The listing builds one solid part. Answer for the finished solid, in the listing's coordinates (mm). Round coordinates to 2 decimals unless told otherwise and drop trailing zeros. Loops run counter-clockwise (first coordinate to the right, second up) from the corner with the lowest first, then second, coordinate; pieces in that order, holes last. Notation, with made-up numbers: (-30.5, 81) -> (-2.5, 81) arc R11 cw to (-2.5, 99) -> close; hole circle Ø11 at (57.5, 35). An arc over 180 degrees is marked (long way). Use a Markdown table: item, result. Add a question column.
Q1. Consider line 1 (Z direction, x = 15.25, y = 19). Determine where the line is inside the solid, lowest interval first.
Q2. For a pull along Y with two mould halves and no side action, classify faces 1 (the flat face through (5, 25, 2)), 2 (the flat face through (9, 0, 1)), 3 (the flat face through (13, 24, 1.9)) as released by +Y, released by -Y, zero draft, split by the parting line, or undercut.
Q3. Section A-A on y = 18.5 is taken. Give the vertices of the cut face in (x, z), then the cut area to 3 significant figures.
from build123d import *

# Parameters (mm, degrees)
SKETCH_1_W          = 18
SKETCH_1_H          = 49
EXTRUDE_1_DEPTH     = 2
CUT_EXTRUDE_1_DEPTH = 0.1


with BuildPart() as part:
    # ｽｹｯﾁ1 → ﾎﾞｽ - 押し出し1 (new body)
    with BuildSketch(Plane.XY):
        with Locations((9, 24.5)):
            Rectangle(SKETCH_1_W, SKETCH_1_H)
    extrude(amount=EXTRUDE_1_DEPTH)

    # ｽｹｯﾁ2 → ｶｯﾄ - 押し出し1 (cut)
    with BuildSketch(Plane.XY.offset(2)):
        Polygon((13.914475661, 36.923076923), (14.348557692, 36.923076923), (14.348557692, 20.4375), (17.096153846, 20.4375), (17.096153846, 17.995192308), (14.348557692, 17.995192308), (14.348557692, 12.5), (12.211538462, 12.5), (12.211538462, 17.995192308), (0.915865385, 17.995192308), align=None)
        Polygon((12.211538462, 20.4375), (12.211538462, 30.779146635), (5.113581731, 20.4375), align=None, mode=Mode.SUBTRACT)
    extrude(amount=-CUT_EXTRUDE_1_DEPTH, mode=Mode.SUBTRACT)


solid = part.part
Checked values:
| question | item | result |
|---|---|---|
| 1 | line 1 | z = 0 to 1.9 |
| 2 | face 1 | zero draft |
| 2 | face 2 | released by -Y |
| 2 | face 3 | undercut |
| 3 | outline | (0, 0) -> (18, 0) -> (18, 2) -> (17.1, 2) -> (17.1, 1.9) -> (1.26, 1.9) -> (1.26, 2) -> (0, 2) -> close |
| 3 | area | 34.4 mm2 |
